Here's how the part is built. I have some questions about the finished solid (model axes, mm). Face numbers are marked on the shaded views. A direction names the side the tool comes from. Give positions to 0.01 mm unless a question says otherwise; leave off trailing zeros. Loops run counter-clockwise (first coordinate to the right, second up) from the corner with the lowest first, then second, coordinate; pieces in that order, holes last. Notation, with made-up numbers: (28.25, -24.75) - (47.25, -24.75) arc R15 cw to (47.25, -12.75) - close; hole circle Ø4 at (84.25, 53). An arc over 180 degrees is marked (long way). Use one line per item in the form item = value.
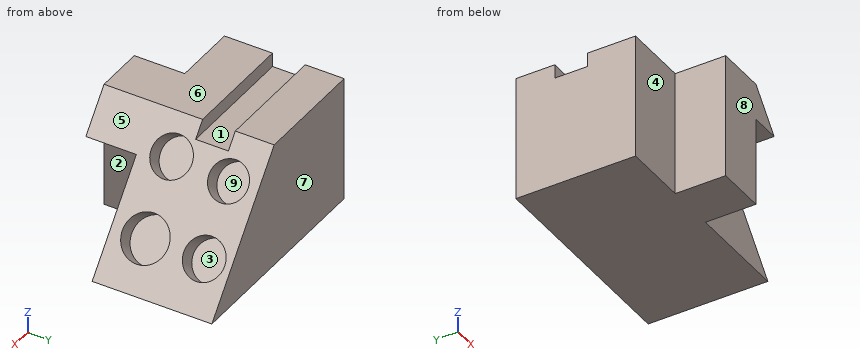
from build123d import *

# Parameters (mm, degrees)
F0_W     = 57.3766939342
F0_H     = 63.22119385
F1_DEPTH = 60.198
F2_R     = 10.2625762698
F2_R_2   = 9.860099692
F2_R_3   = 10.2778616748
F2_R_4   = 11.6361119367
F3_DEPTH = 9.906
F5_DEPTH = 25.4
F6_W     = 16.4541173726
F6_H     = 7.0413090289
F7_DEPTH = 208.28


with BuildPart() as f1:
    # F0 (on Front) → F1 (new body)
    with BuildSketch(Plane.XZ):
        with Locations((-28.6883469671, 31.610596925)):
            Rectangle(F0_W, F0_H)
        Polygon((0, 63.22119385), (0, 0), (51.1963777244, 0), align=None)
    extrude(amount=F1_DEPTH)

    # F2 (on face) → F3 (cut)
    with BuildSketch(Plane(origin=(30.9199380754, 0, 25.0388949105), x_dir=(0, 1, 0), z_dir=(0.7771407648, 0, 0.6293268083))):
        with Locations((-44.1004633904, 29.6253170818)):
            Circle(F2_R)
        with Locations((-14.7637147456, 27.8175938874)):
            Circle(F2_R_2)
        with Locations((-13.5386008769, -7.013282273)):
            Circle(F2_R_3)
        with Locations((-43.0233776569, -7.2796405293)):
            Circle(F2_R_4)
    extrude(amount=-F3_DEPTH, mode=Mode.SUBTRACT)

    # F4 (on face) → F5 (join)
    with BuildSketch(Plane.XZ.offset(60.198)):
        Polygon((0, 63.22119385), (-24.8047709465, 63.22119385), (-24.8047709465, 0), (0, 0), (0, 44.7936064249), align=None)
        Polygon((14.9226180164, 44.7936064249), (0, 63.22119385), (0, 44.7936064249), align=None)
    extrude(amount=F5_DEPTH)

    # F6 (on face) → F7 (cut)
    with BuildSketch(Plane(origin=(-57.3766939342, 0, 0), x_dir=(0, -1, 0), z_dir=(-1, 0, 0))):
        with Locations((27.7932761237, 59.7005393356)):
            Rectangle(F6_W, F6_H)
    extrude(amount=-F7_DEPTH, mode=Mode.SUBTRACT)


solid = f1.part
(1) If we section it at D-D (y = -48): List the corners of the cut face in (x, z) for me, plus the area to 3 significant figures.
Geometry says:
outline = (-57.38, 0) - (51.2, 0) - (42.12, 11.21) - (34.42, 4.97) - (21.18, 21.32) - (28.88, 27.56) - (18.25, 40.68) - (10.55, 34.45) - (-1.4, 49.21) - (6.3, 55.44) - (0, 63.22) - (-57.38, 63.22) - close
area = 4,850 mm²
(2) If we section it at C-C (z = 38.5): Give the number of separate pieces and of enclosed holes in the cut face, plus the area to 3 significant figures.
Geometry says:
separate_pieces = 1
enclosed_holes = 2
area = 5,000 mm²
(3) For the marked faces 1, 2, 3, 4 and 5, which set-ups out of +Z, -Z, +X, -X, +Y, -Y let a thin tool reach every point of the face, with its end or its side?
Geometry says:
face_1 = +Z, +X, -X
face_2 = -Z, +X, -Y
face_3 = none
face_4 = +Z, -Z, -X, -Y
face_5 = +Z, +X, +Y, -Y
(4) If I drill on probe 1 along Z at (x, y) = (4, -30); probe 2 along X at (y, z) = (-16, 35); probe 3 along X at (y, z) = (-9, 8), over which ranges is the centre line in solid material (lowest first)?
Geometry says:
probe_1 = 0 to 56.18
probe_2 = -57.38 to 10.11, 14.56 to 22.85
probe_3 = -57.38 to 31.97, 35.68 to 44.72
(5) For P1, Ø3, axis at x = -40, z = 33.5, coming from the -Y side; P2, Ø12, axis at y = -17, z = 38, coming from the +X side; P3, Ø12, axis at x = 36, y = -68.5, coming from the -Z side; P4, Ø4.5, axis at x = 8.5, y = -74, coming from the -Z side, each with a flat end and sliding along its axis, tell me the tip position at first contact or that it passes through.
Geometry says:
P1 = -60.2
P2 = 25.28
P3 = through
P4 = 44.79
(6) Thinking about a two-plate mould opening in Y: for the marked faces 6, 7, 8 and 9, which applies, pulls with the +Y half, pulls with the -Y half, needs draft (parallel to the pull), parting line crosses it, or undercut?
Geometry says:
face_6 = needs draft
face_7 = pulls with the +Y half
face_8 = pulls with the -Y half
face_9 = undercut
(7) If we section it at A-A (x = -19): List the corners of the cut face in (y, z) for me, plus the area to 3 significant figures.
Geometry says:
outline = (-85.6, 0) - (0, 0) - (0, 63.22) - (-19.57, 63.22) - (-19.57, 56.18) - (-36.02, 56.18) - (-36.02, 63.22) - (-85.6, 63.22) - close
area = 5,300 mm²
(8) If we section it at B-B (y = -68): List the corners of the cut face in (x, z) for me, plus the area to 3 significant figures.
Geometry says:
outline = (-24.8, 0) - (0, 0) - (0, 44.79) - (14.92, 44.79) - (0, 63.22) - (-24.8, 63.22) - close
area = 1,710 mm²
